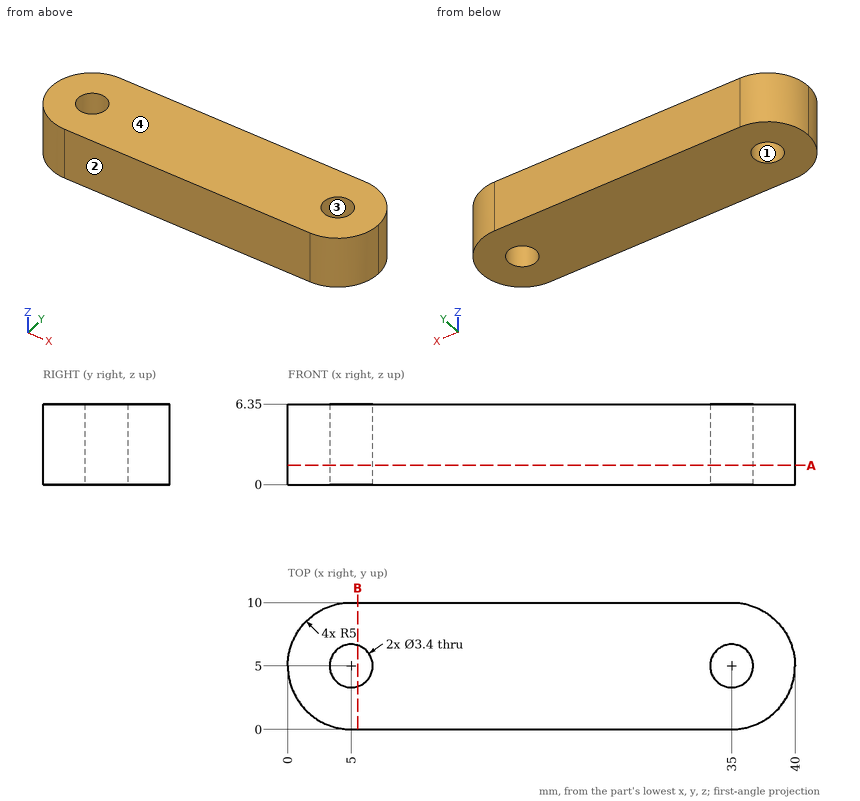
Could you check a few things on this drawing? It's one solid part, dimensions in mm from its lowest x, y, z. Coordinates: 2 decimals unless noted, no trailing zeros. Order: outer loops, then holes, each group sorted by start corner. A loop starts at its lowest first (then second) coordinate and runs counter-clockwise, first axis right, second up. Notation, with made-up numbers: (-13.75, 28.25) - (-6.75, 28.25) arc R25 ccw to (-6.75, 40.25) - close; hole circle Ø7 at (-14, -1). An arc over 180 degrees is marked (long way). One line per question, with ' | ' between items.
(1) If I drill on L1, parallel to Y at x = 5, z = 2.75; L2, parallel to X at y = 6, z = 1.25 (1 decimal); L3, parallel to Y at x = 4, z = 2.75 (1 decimal), over which ranges is the centre line in solid material (lowest first)?
Report:
L1: y = 0 to 3.3, 6.7 to 10 | L2: x = 0.1 to 3.6, 6.4 to 33.6, 36.4 to 39.9 | L3: y = 0.1 to 3.6, 6.4 to 9.9
(2) If we mould it in two halves opening along Y, with no side actions, what happens to the marked faces 1, 2, 3 and 4? For each: pulls with the +Y half, pulls with the -Y half, needs draft (parallel to the pull), parting line crosses it, or undercut.
Report:
face 1: undercut | face 2: pulls with the -Y half | face 3: undercut | face 4: needs draft
(3) Suppose I cut it at B-B on x = 5.5. List the corners of the cut face in (y, z) for me (3 decimals), and give its area (3 significant figures).
Report:
outline: (0, 0) - (3.375, 0) - (3.375, 6.35) - (0, 6.35) - close; (6.625, 0) - (10, 0) - (10, 6.35) - (6.625, 6.35) - close | area: 42.9 mm2
(4) Suppose I cut it at A-A on z = 1.5. State how many separate pieces and enclosed holes the cut face has, and give its area (3 significant figures).
Report:
separate pieces: 1 | enclosed holes: 2 | area: 360 mm2
